```python
from build123d import *

# Parameters (mm, degrees)
SKETCH5_R          = 2.499999953
CUT_EXTRUDE1_DEPTH = 13.979399746


with BuildPart() as part:
    # Sketch3 → Revolve1 (revolve)
    with BuildSketch(Plane.XY):
        Polygon((12.979399746, 2.999999969), (12.979399746, 2.499999953), (12.979399746, 0), (6.009399716, 0), (6.009399716, 2.499999953), (6.009399716, 5.999999938), (9.97939965, 5.999999938), (10.879399628, 5.999999938), (10.879399628, 5.450000022), (11.979399714, 5.450000022), (11.979399714, 5.999999938), (12.979399746, 5.999999938), align=None)
    revolve(axis=Axis((6.009399716, 0, 0), (1, 0, 0)))

    # Sketch5 → Cut-Extrude1 (cut, through all)
    with BuildSketch(Plane(origin=(0, 0, 0), x_dir=(0, 0, -1), z_dir=(1, 0, 0))):
        with Locations((1.5875, 0)):
            Circle(SKETCH5_R)
    extrude(amount=CUT_EXTRUDE1_DEPTH, mode=Mode.SUBTRACT)


solid = part.part
```
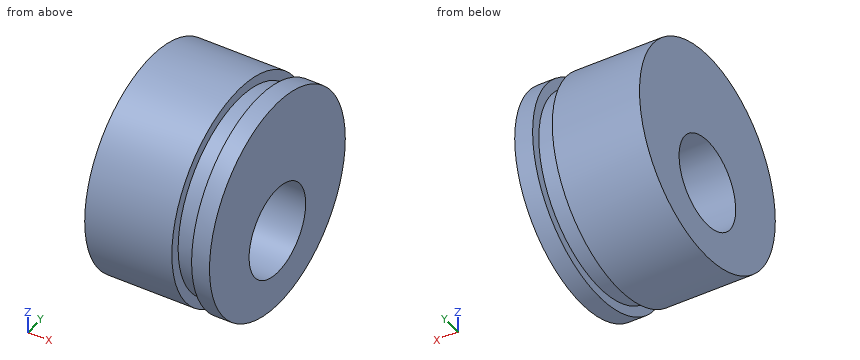
CAD build for the part. Positions are in the model's coordinates, mm. Give positions to 0.01 mm unless a question says otherwise; leave off trailing zeros. Order: outer loops, then holes, each group sorted by start corner. A loop starts at its lowest first (then second) coordinate and runs counter-clockwise, first axis right, second up.
(1) Saw through at D-D, the plane y = -3.75. Give the cut face in (x, z).
(2) Saw through at C-C, the plane x = 11.5. Give the cut face in (y, z), then the cut area to 3 significant figures.
(3) Saw through at A-A, the plane z = 0. Give the cut face in (x, y).
(4) Flat gauge pins, fed straight in: pin 1 (2 mm diameter, centred on x = 8.5, y = 3.5, fed in from +Z); pin 2 (2 mm diameter, centred on x = 10.5, y = 2.5, fed in from +Z); pin 3 (1.5 mm diameter, centred on x = 9, y = 3.5, fed in from +Z). Where does each tip first touch, or does it go through?
(5) Saw through at B-B, the plane y = -1.5. Give the cut face in (x, z).
(6) Drill centre lines: L1, parallel to Z at x = 10, y = 0; L2, parallel to X at y = 1.75, z = 5.25; L3, parallel to Z at x = 11.25, y = 0. Where is each one in solid material? Low to high.
Results found:
1. outline: (6.01, -4.68) - (10.88, -4.68) - (10.88, -3.95) - (11.98, -3.95) - (11.98, -4.68) - (12.98, -4.68) - (12.98, 4.68) - (11.98, 4.68) - (11.98, 3.95) - (10.88, 3.95) - (10.88, 4.68) - (6.01, 4.68) - close
2. outline: circle Ø10.9 at (0, 0); hole circle Ø5 at (0, -1.59)
2. area: 73.7 mm2
3. outline: (6.01, -6) - (10.88, -6) - (10.88, -5.45) - (11.98, -5.45) - (11.98, -6) - (12.98, -6) - (12.98, -1.93) - (6.01, -1.93) - close; (6.01, 1.93) - (12.98, 1.93) - (12.98, 6) - (11.98, 6) - (11.98, 5.45) - (10.88, 5.45) - (10.88, 6) - (6.01, 6) - close
4. pin 1: stops at z = 5.45
4. pin 2: stops at z = 5.81
4. pin 3: stops at z = 5.33
5. outline: (6.01, -5.81) - (10.88, -5.81) - (10.88, -5.24) - (11.98, -5.24) - (11.98, -5.81) - (12.98, -5.81) - (12.98, -3.59) - (6.01, -3.59) - close; (6.01, 0.41) - (12.98, 0.41) - (12.98, 5.81) - (11.98, 5.81) - (11.98, 5.24) - (10.88, 5.24) - (10.88, 5.81) - (6.01, 5.81) - close
6. L1: z = -6 to -4.09, 0.91 to 6
6. L2: x = 6.01 to 10.88, 11.98 to 12.98
6. L3: z = -5.45 to -4.09, 0.91 to 5.45
